```python
from build123d import *

# Parameters (mm, degrees)
EXTRUDE_1_DEPTH = 4


with BuildPart() as part:
    # 草图1 → 凸台-拉伸1 (new body)
    with BuildSketch(Plane.XY):
        with BuildLine():
            Line((0, 9.65), (0, 14))
            ThreePointArc((0, 14), (-14, 0), (0, -14))
            Line((0, -14), (0, -9.65))
            ThreePointArc((0, -9.65), (-1.225409689, -9.104930357), (-1.641202867, -7.82984375))
            ThreePointArc((-1.641202867, -7.82984375), (-5.656854249, -5.656854249), (-7.82984375, -1.641202867))
            ThreePointArc((-7.82984375, -1.641202867), (-9.65, 0), (-7.82984375, 1.641202867))
            ThreePointArc((-7.82984375, 1.641202867), (-5.656854249, 5.656854249), (-1.641202867, 7.82984375))
            ThreePointArc((-1.641202867, 7.82984375), (-1.225409689, 9.104930357), (0, 9.65))
        make_face()
        with BuildLine():
            ThreePointArc((0, 6.35), (-1.104930357, 6.774590311), (-1.641202867, 7.82984375))
            ThreePointArc((-1.641202867, 7.82984375), (-5.656854249, 5.656854249), (-7.82984375, 1.641202867))
            ThreePointArc((-7.82984375, 1.641202867), (-6.774590311, 1.104930357), (-6.35, 0))
            ThreePointArc((-6.35, 0), (-6.774590311, -1.104930357), (-7.82984375, -1.641202867))
            ThreePointArc((-7.82984375, -1.641202867), (-5.656854249, -5.656854249), (-1.641202867, -7.82984375))
            ThreePointArc((-1.641202867, -7.82984375), (-1.104930357, -6.774590311), (0, -6.35))
            Line((0, -6.35), (0, -5.2))
            ThreePointArc((0, -5.2), (-5.2, 0), (0, 5.2))
            Line((0, 5.2), (0, 6.35))
        make_face()
        with BuildLine():
            ThreePointArc((1.641202867, 7.82984375), (1.104930357, 6.774590311), (0, 6.35))
            Line((0, 6.35), (0, 5.2))
            ThreePointArc((0, 5.2), (3.676955262, 3.676955262), (5.2, 0))
            ThreePointArc((5.2, 0), (3.676955262, -3.676955262), (0, -5.2))
            Line((0, -5.2), (0, -6.35))
            ThreePointArc((0, -6.35), (1.104930357, -6.774590311), (1.641202867, -7.82984375))
            ThreePointArc((1.641202867, -7.82984375), (5.656854249, -5.656854249), (7.82984375, -1.641202867))
            ThreePointArc((7.82984375, -1.641202867), (6.35, 0), (7.82984375, 1.641202867))
            ThreePointArc((7.82984375, 1.641202867), (5.656854249, 5.656854249), (1.641202867, 7.82984375))
        make_face()
        with BuildLine():
            ThreePointArc((14, 0), (9.899494937, 9.899494937), (0, 14))
            Line((0, 14), (0, 9.65))
            ThreePointArc((0, 9.65), (1.166726189, 9.166726189), (1.65, 8))
            ThreePointArc((1.65, 8), (1.647799249, 7.914808247), (1.641202867, 7.82984375))
            ThreePointArc((1.641202867, 7.82984375), (5.656854249, 5.656854249), (7.82984375, 1.641202867))
            ThreePointArc((7.82984375, 1.641202867), (9.104930357, 1.225409689), (9.65, 0))
            ThreePointArc((9.65, 0), (9.104930357, -1.225409689), (7.82984375, -1.641202867))
            ThreePointArc((7.82984375, -1.641202867), (5.656854249, -5.656854249), (1.641202867, -7.82984375))
            ThreePointArc((1.641202867, -7.82984375), (1.647799249, -7.914808247), (1.65, -8))
            ThreePointArc((1.65, -8), (1.166726189, -9.166726189), (0, -9.65))
            Line((0, -9.65), (0, -14))
            ThreePointArc((0, -14), (9.899494937, -9.899494937), (14, 0))
        make_face()
        with BuildLine():
            ThreePointArc((94, 0), (89.899494937, 9.899494937), (80, 14))
            Line((80, 14), (80, 9.65))
            ThreePointArc((80, 9.65), (81.166726189, 9.166726189), (81.65, 8))
            ThreePointArc((81.65, 8), (81.647799249, 7.914808247), (81.641202867, 7.82984375))
            ThreePointArc((81.641202867, 7.82984375), (85.656854249, 5.656854249), (87.82984375, 1.641202867))
            ThreePointArc((87.82984375, 1.641202867), (89.104930357, 1.225409689), (89.65, 0))
            ThreePointArc((89.65, 0), (89.104930357, -1.225409689), (87.82984375, -1.641202867))
            ThreePointArc((87.82984375, -1.641202867), (85.656854249, -5.656854249), (81.641202867, -7.82984375))
            ThreePointArc((81.641202867, -7.82984375), (81.647799249, -7.914808247), (81.65, -8))
            ThreePointArc((81.65, -8), (81.166726189, -9.166726189), (80, -9.65))
            Line((80, -9.65), (80, -14))
            ThreePointArc((80, -14), (89.899494937, -9.899494937), (94, 0))
        make_face()
        with BuildLine():
            Line((80, 9.65), (80, 14))
            ThreePointArc((80, 14), (66, 0), (80, -14))
            Line((80, -14), (80, -9.65))
            ThreePointArc((80, -9.65), (78.774590311, -9.104930357), (78.358797133, -7.82984375))
            ThreePointArc((78.358797133, -7.82984375), (74.343145751, -5.656854249), (72.17015625, -1.641202867))
            ThreePointArc((72.17015625, -1.641202867), (70.35, 0), (72.17015625, 1.641202867))
            ThreePointArc((72.17015625, 1.641202867), (74.343145751, 5.656854249), (78.358797133, 7.82984375))
            ThreePointArc((78.358797133, 7.82984375), (78.774590311, 9.104930357), (80, 9.65))
        make_face()
        with BuildLine():
            ThreePointArc((80, 6.35), (78.895069643, 6.774590311), (78.358797133, 7.82984375))
            ThreePointArc((78.358797133, 7.82984375), (74.343145751, 5.656854249), (72.17015625, 1.641202867))
            ThreePointArc((72.17015625, 1.641202867), (73.225409689, 1.104930357), (73.65, 0))
            ThreePointArc((73.65, 0), (73.225409689, -1.104930357), (72.17015625, -1.641202867))
            ThreePointArc((72.17015625, -1.641202867), (74.343145751, -5.656854249), (78.358797133, -7.82984375))
            ThreePointArc((78.358797133, -7.82984375), (78.895069643, -6.774590311), (80, -6.35))
            Line((80, -6.35), (80, -5.3))
            ThreePointArc((80, -5.3), (74.7, 0), (80, 5.3))
            Line((80, 5.3), (80, 6.35))
        make_face()
        with BuildLine():
            ThreePointArc((81.641202867, 7.82984375), (81.104930357, 6.774590311), (80, 6.35))
            Line((80, 6.35), (80, 5.3))
            ThreePointArc((80, 5.3), (83.74766594, 3.74766594), (85.3, 0))
            ThreePointArc((85.3, 0), (83.74766594, -3.74766594), (80, -5.3))
            Line((80, -5.3), (80, -6.35))
            ThreePointArc((80, -6.35), (81.104930357, -6.774590311), (81.641202867, -7.82984375))
            ThreePointArc((81.641202867, -7.82984375), (85.656854249, -5.656854249), (87.82984375, -1.641202867))
            ThreePointArc((87.82984375, -1.641202867), (86.35, 0), (87.82984375, 1.641202867))
            ThreePointArc((87.82984375, 1.641202867), (85.656854249, 5.656854249), (81.641202867, 7.82984375))
        make_face()
        with BuildLine():
            Line((80, 14), (0, 14))
            ThreePointArc((0, 14), (9.899494937, 9.899494937), (14, 0))
            ThreePointArc((14, 0), (9.899494937, -9.899494937), (0, -14))
            Line((0, -14), (80, -14))
            ThreePointArc((80, -14), (66, 0), (80, 14))
        make_face()
    extrude(amount=EXTRUDE_1_DEPTH)


solid = part.part
```
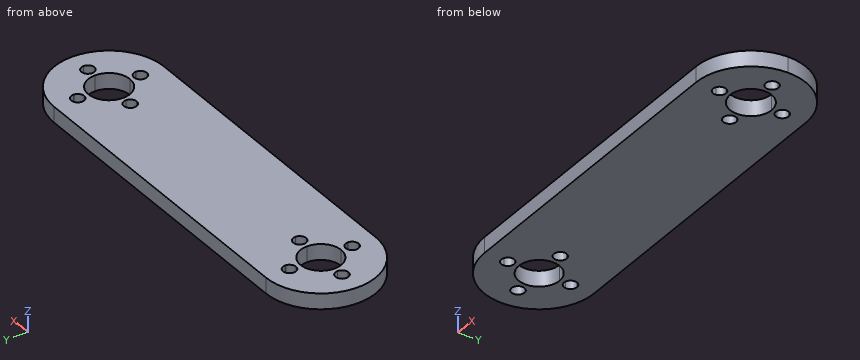
CAD build for the part. Positions are in the model's coordinates, mm. Coordinates: 2 decimals unless noted, no trailing zeros. Use CSV: the item, a comma, the result in double quotes. Start each with the question number.
Q1. Drop a flat-ended pin along its axis: P1, Ø2, axis at y = 9, z = 3, coming from the -X side. Give the stop position or say it passes through.
Q2. Probe probe 1 along X at (y, z) = (9.25, 3.55); probe 2 along X at (y, z) = (-6.5, 3.05); probe 3 along Y at (x, z) = (72, 1.95). List the from-to ranges inside material, lowest first. Write a range as from..to.
Q3. Cut at A-A, the plane z = 2.4. State how many separate pieces and enclosed holes the cut face has, then the cut area to 3 significant figures.
Here are the results:
1,P1,"x = -11.49"
2,probe 1,"-10.51..-1.08, 1.08..78.92, 81.08..90.51"
2,probe 2,"-12.4..-0.69, 0.69..79.31, 80.69..92.4"
2,probe 3,"-14..-1.65, 1.65..14"
3,separate pieces,"1"
3,enclosed holes,"10"
3,area,"2,610 mm2"
